Can you work these out from the model? Positions are in its coordinate system, mm. Coordinates: 2 decimals unless noted, no trailing zeros. Order: outer loops, then holes, each group sorted by start corner. A loop starts at its lowest first (then second) coordinate and runs counter-clockwise, first axis right, second up. Notation, with made-up numbers: (-27, 48) -> (-9, 48) arc R20 cw to (-9, 82) -> close; hole circle Ø7 at (42, 14). An arc over 180 degrees is marked (long way). Answer in a Markdown table with one row per item. Add a question column.
1. Imagine slicing it at A-A on z = 0. Write out the boundary of the cut face in (x, y) (3 decimals), plus the area to 3 significant figures.
2. Imagine slicing it at B-B on x = -20. Write out the boundary of the cut face in (y, z), plus the area to 3 significant figures.
3. Will this pin go through, and if not, where does the flat tip stop? pin 1 (1.3 mm diameter, centred on x = 20, z = 7.5, fed in from +Y).
4. We'd pull the mould along Z, two halves only. Please class faces 1 (the face through (21.1, 0.5, -7.5)), 2 (the face through (-0.2, 0.5, -12.875)), 3 (the face through (25.12, 0.49, -0.28)): pulls with the +Z half, pulls with the -Z half, needs draft (parallel to the pull), parting line crosses it, or undercut.
5. If I drill on line 1 along X through (y, z) = (0.35, -7.25); line 2 along Z through (x, y) = (-20, 0.8); line 3 along X through (y, z) = (0.85, 7.5), over which ranges is the centre line in solid material (lowest first)? Write a range as [from, to].
6. Imagine slicing it at D-D on x = 19.5. Write out the boundary of the cut face in (y, z), plus the area to 3 significant figures.
7. Imagine slicing it at C-C on y = 0.2. State how many separate pieces and enclosed holes the cut face has, plus the area to 3 significant figures.
from build123d import *

# Parameters (mm, degrees)
BOSS_EXTRUDE1_DEPTH      = 1
SKETCH2_R                = 11
CUT_EXTRUDE1_DEPTH       = 10.811106589
CUT_EXTRUDE1_DEPTH_BACK  = 27.428115947
M2_CLEARANCE_HOLE1_D     = 2.2
M2_CLEARANCE_HOLE1_DEPTH = 1


with BuildPart() as part:
    # Sketch1 → Boss-Extrude1 (new body)
    with BuildSketch(Plane(origin=(0, 0, 0), x_dir=(1, 0, 0), z_dir=(0, 1, 0))):
        with BuildLine():
            Line((-12.25, 12.875), (12.25, 12.875))
            ThreePointArc((12.25, 12.875), (25.125, 0), (12.25, -12.875))
            Line((12.25, -12.875), (-12.25, -12.875))
            ThreePointArc((-12.25, -12.875), (-25.125, 0), (-12.25, 12.875))
        make_face()
    extrude(amount=BOSS_EXTRUDE1_DEPTH)

    # Sketch2 → Cut-Extrude1 (cut, two sides)
    with BuildSketch(Plane(origin=(6.125, 6.125, 0), x_dir=(0, 0, 1), z_dir=(0.707106781, 0.707106781, 0))) as cut_extrude1_sk:
        with Locations((0, -0.707106781)):
            Circle(SKETCH2_R)
    extrude(amount=CUT_EXTRUDE1_DEPTH, mode=Mode.SUBTRACT)
    extrude(cut_extrude1_sk.sketch, amount=-CUT_EXTRUDE1_DEPTH_BACK, mode=Mode.SUBTRACT)

    # M2 Clearance Hole1
    with Locations(Plane(origin=(0, 1, 0), x_dir=(1, 0, 0), z_dir=(0, 1, 0))):
        with Locations((-20, 7.5), (-20, -7.5), (20, -7.5), (20, 7.5)):
            Hole(M2_CLEARANCE_HOLE1_D / 2, depth=M2_CLEARANCE_HOLE1_DEPTH)


solid = part.part
Answers follow:
| question | item | result |
|---|---|---|
| 1 | outline | (-25.125, 0) -> (-16.556, 0) -> (-15.556, 1) -> (-25.125, 1) -> close; (14.556, 0) -> (25.125, 0) -> (25.125, 1) -> (15.556, 1) -> close |
| 1 | area | 19.1 mm² |
| 2 | outline | (0, -10.28) -> (1, -10.28) -> (1, -8.6) -> (0, -8.6) -> close; (0, -6.4) -> (1, -6.4) -> (1, 6.4) -> (0, 6.4) -> close; (0, 8.6) -> (1, 8.6) -> (1, 10.28) -> (0, 10.28) -> close |
| 2 | area | 16.2 mm² |
| 3 | pin 1 | passes through |
| 4 | face 1 | undercut |
| 4 | face 2 | pulls with the -Z half |
| 4 | face 3 | parting line crosses it |
| 5 | line 1 | x = [-22.89, -21.07], [-18.93, -12.35], [11.05, 18.93], [21.07, 22.89] |
| 5 | line 2 | z = [-10.28, -8.6], [-6.4, 6.4], [8.6, 10.28] |
| 5 | line 3 | x = [-22.71, -21.1], [-18.9, -11.53], [11.23, 18.9], [21.1, 22.71] |
| 6 | outline | (0, -10.64) -> (1, -10.64) -> (1, -8.48) -> (0, -8.48) -> close; (0, -6.52) -> (1, -6.52) -> (1, 6.52) -> (0, 6.52) -> close; (0, 8.48) -> (1, 8.48) -> (1, 10.64) -> (0, 10.64) -> close |
| 6 | area | 17.4 mm² |
| 7 | separate pieces | 1 |
| 7 | enclosed holes | 5 |
| 7 | area | 599 mm² |
